from build123d import *

# Parameters (mm, degrees)
F0_R      = 40
F0_R_2    = 37.75
F1_DEPTH  = 15
F2_DEPTH  = 10
F0_R_3    = 25
F3_DEPTH  = 1.25
F0_R_4    = 22.5
F4_DEPTH  = 30
F5_DEPTH  = 1.25
F7_R      = 5
F8_DEPTH  = 39
F9_R      = 5
F11_R     = 6.5
F11_R_2   = 5
F12_DEPTH = 17
F13_DEPTH = 10


with BuildPart() as f1:
    # F0 (on Front) → F1 (new body)
    with BuildSketch(Plane.XZ):
        with Locations((-137.480571866, 0)):
            Circle(F0_R)
        with Locations((-137.480571866, 0)):
            Circle(F0_R_2, mode=Mode.SUBTRACT)
    extrude(amount=F1_DEPTH)

    # F2 (add): a face of the model
    f2_faces = [f1.faces().sort_by_distance(p)[0] for p in [
        (-176.3492010161, 0, 0),
    ]]
    extrude(f2_faces, amount=F2_DEPTH)

    # F0 (on Front) → F3 (join, symmetric)
    with BuildSketch(Plane.XZ):
        with Locations((-137.480571866, 0)):
            Circle(F0_R_2)
        with Locations((-137.480571866, 0)):
            Circle(F0_R_3, mode=Mode.SUBTRACT)
    extrude(amount=F3_DEPTH, both=True)

    # F0 (on Front) → F4 (join)
    with BuildSketch(Plane.XZ):
        with Locations((-137.480571866, 0)):
            Circle(F0_R_3)
        with Locations((-137.480571866, 0)):
            Circle(F0_R_4, mode=Mode.SUBTRACT)
    extrude(amount=F4_DEPTH)

    # F5 (add): a face of the model
    f5_faces = [f1.faces().sort_by_distance(p)[0] for p in [
        (-161.7734650848, 0, 0),
    ]]
    extrude(f5_faces, amount=F5_DEPTH)

    # F7 (on offset) → F8 (cut)
    with BuildSketch(Plane.YZ.offset(-107.4)):
        with Locations((-5.8384072036, 0)):
            Circle(F7_R)
    extrude(amount=F8_DEPTH, mode=Mode.SUBTRACT)

    # F9
    f9_edges = [f1.edges().sort_by_distance(p)[0] for p in [
        (-103.59144, -1.25, 1.986585),
        (-103.59144, -1.25, -1.986585),
    ]]
    fillet(f9_edges, radius=F9_R)

    # F11 (on offset) → F12 (join)
    with BuildSketch(Plane.YZ.offset(-98.7)):
        with Locations((-5.8384072036, 0)):
            Circle(F11_R)
        with Locations((-5.8384072036, 0)):
            Circle(F11_R_2, mode=Mode.SUBTRACT)
    extrude(amount=F12_DEPTH)

    # F11 (on offset) → F13 (join)
    with BuildSketch(Plane.YZ.offset(-98.7)):
        with Locations((-5.8384072036, 0)):
            Circle(F11_R)
        with Locations((-5.8384072036, 0)):
            Circle(F11_R_2, mode=Mode.SUBTRACT)
    extrude(amount=F13_DEPTH)


solid = f1.part
Design review of the part built by this model. Coordinates are the model's own, in mm. A direction names the side the tool comes from. Round coordinates to 2 decimals unless told otherwise and drop trailing zeros. Write each loop counter-clockwise with the first axis right and the second up, starting at its lowest first coordinate (ties: lowest second). Pieces come first, ordered by that corner, then holes.
Item 1: Consider section D-D on y = -20.5. Give the boundary of the cut face in (x, z), and give its area (3 significant figures).
Item 2: For pin 1 Ø6 at (x, z) = (-154, -6.5) entering from +Y; pin 2 Ø8 at (y, z) = (-5.84, 0) entering from +X; pin 3 Ø8 at (x, y) = (-161.5, -23.5) entering from -Z; pin 4 Ø3 at (x, y) = (-127, -2.5) entering from +Z, all flat-tipped, find the tip position at first contact; note any pin that passes through.
Item 3: Consider section B-B on z = 0. Give the boundary of the cut face in (x, y), and give its area (3 significant figures).
Item 4: Draft analysis for pull direction X (two halves, no side actions). For faces 1 (the flat face through (-108, 10, 24)), 2 (the cylindrical face through (-101.474, 5.564, 11.339)), 3 (the cylindrical face through (-99.328, -2.675, 12.015)), state which applies: released by +X, released by -X, zero draft, split by the parting line, or undercut.
Item 5: Consider section A-A on y = -9. Give the boundary of the cut face in (x, z).
Item 6: Wall thickness on L1, parallel to Y at x = -89, z = 0; L2, parallel to X at y = -3.5, z = 18; L3, parallel to Z at x = -137, y = 8: over which ranges is each line inside the solid? List them lowest first.
Item 7: Consider section C-C on x = -121.5. Give the boundary of the cut face in (y, z), and give its area (3 significant figures).
Item 8: For faces 4 (the cylindrical face through (-89.97, -10.997, -3.955)), 5 (the cylindrical face through (-113.635, -15.424, 7.509)), 6 (the flat face through (-81.7, -2, -4)), 7 (the flat face through (-121, 1.25, -16)), list the 3-axis set-ups (+Z, -Z, +X, -X, +Y, -Y) from which the entire face can be reached by the end or side of a thin tool; tool diameter is ignored.
Check values:
1. outline: circle Ø50 at (-137.48, 0); hole circle Ø45 at (-137.48, 0)
1. area: 373 mm2
2. pin 1: passes through
2. pin 2: stops at x = -112.48
2. pin 3: stops at z = -14.97
2. pin 4: stops at z = 38.98
3. outline: (-177.48, -15) - (-175.23, -15) - (-175.23, -1.25) - (-162.48, -1.25) - (-162.48, -30) - (-159.98, -30) - (-159.98, 1.25) - (-175.23, 1.25) - (-175.23, 10) - (-177.48, 10) - close; (-114.98, -30) - (-112.48, -30) - (-112.48, -1.25) - (-107.4, -1.25) - (-107.4, -0.84) - (-81.7, -0.84) - (-81.7, 0.66) - (-97.48, 0.66) - (-97.48, 10) - (-99.73, 10) - (-99.73, 1.25) - (-114.98, 1.25) - close; (-99.73, -15) - (-97.48, -15) - (-97.48, -12.34) - (-81.7, -12.34) - (-81.7, -10.84) - (-99.73, -10.84) - close
3. area: 354 mm2
4. face 1: zero draft
4. face 2: undercut
4. face 3: split by the parting line
5. outline: circle Ø50 at (-137.48, 0); (-99.93, -3.87) arc R37.75 cw (long way) to (-99.93, 3.87) - (-81.7, 3.87) - (-81.7, 5.68) - (-97.89, 5.68) arc R40 ccw (long way) to (-97.89, -5.68) - (-81.7, -5.68) - (-81.7, -3.87) - close; hole circle Ø45 at (-137.48, 0)
6. L1: y = -12.34 to -10.84, -0.84 to 0.66
6. L2: x = -173.2 to -170.66, -154.83 to -150.98, -123.98 to -120.13, -104.3 to -101.76
6. L3: z = -40 to -37.75, 37.75 to 40
7. outline: (-30, -19.23) - (-1.25, -19.23) - (-1.25, -34.2) - (-15, -34.2) - (-15, -36.67) - (10, -36.67) - (10, -34.2) - (1.25, -34.2) - (1.25, -15.84) - (-30, -15.84) - close; (-30, 15.84) - (1.25, 15.84) - (1.25, 34.2) - (10, 34.2) - (10, 36.67) - (-15, 36.67) - (-15, 34.2) - (-1.25, 34.2) - (-1.25, 19.23) - (-30, 19.23) - close
7. area: 410 mm2
8. face 4: +X
8. face 5: -Y
8. face 6: +Z, -Z, +X, +Y, -Y
8. face 7: +Y
